The listing builds one solid part. Answer for the finished solid, in the listing's coordinates (mm). Give positions to 0.01 mm unless a question says otherwise; leave off trailing zeros. Order: outer loops, then holes, each group sorted by start corner. A loop starts at its lowest first (then second) coordinate and runs counter-clockwise, first axis right, second up.
```python
from build123d import *

# Parameters (mm, degrees)
ESBO_O1_W                = 152
ESBO_O1_H                = 60
RESSALTO_EXTRUS_O2_DEPTH = 6


with BuildPart() as part:
    # Esboço1 → Ressalto-extrusão2 (new body)
    with BuildSketch(Plane.XY):
        Rectangle(ESBO_O1_W, ESBO_O1_H)
        with BuildLine():
            Line((45, -16), (-45, -16))
            ThreePointArc((-45, -16), (-52.071067812, -13.071067812), (-55, -6))
            Line((-55, -6), (-55, 6))
            ThreePointArc((-55, 6), (-52.071067812, 13.071067812), (-45, 16))
            Line((-45, 16), (45, 16))
            ThreePointArc((45, 16), (52.071067812, 13.071067812), (55, 6))
            Line((55, 6), (55, -6))
            ThreePointArc((55, -6), (52.071067812, -13.071067812), (45, -16))
        make_face(mode=Mode.SUBTRACT)
    extrude(amount=RESSALTO_EXTRUS_O2_DEPTH)


solid = part.part
```
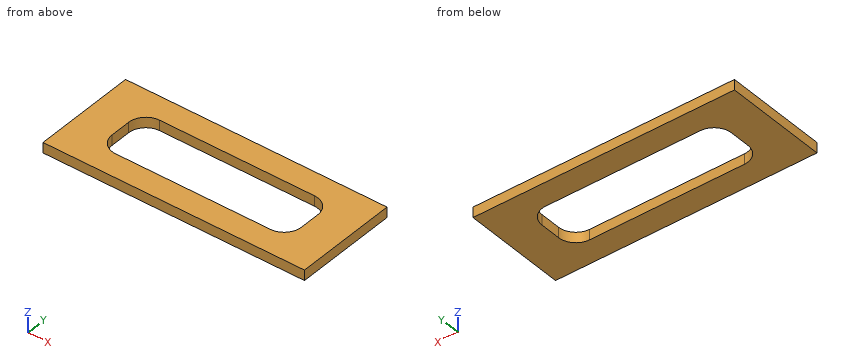
1) Find section C-C (x = 35.5). Write down the section's boundary in (y, z).
Geometry says:
outline: (-30, 0) - (-16, 0) - (-16, 6) - (-30, 6) - close; (16, 0) - (30, 0) - (30, 6) - (16, 6) - close
2) Find section B-B (y = -12). Write down the section's boundary in (x, z), then the cut area to 3 significant figures.
Geometry says:
outline: (-76, 0) - (-53, 0) - (-53, 6) - (-76, 6) - close; (53, 0) - (76, 0) - (76, 6) - (53, 6) - close
area: 276 mm2
3) Straight lines are drawn through the part: probe 1 along Y at (x, z) = (-28.5, 5.65); probe 2 along X at (y, z) = (-4, 4.35); probe 3 along X at (y, z) = (-8, 5.8). For each, find the intervals that lie inside material, in ascending order.
Geometry says:
probe 1: y = -30 to -16, 16 to 30
probe 2: x = -76 to -55, 55 to 76
probe 3: x = -76 to -54.8, 54.8 to 76
4) Find section A-A (z = 4.6). Write down the section's boundary in (x, y).
Geometry says:
outline: (-76, -30) - (76, -30) - (76, 30) - (-76, 30) - close; hole (-55, -6) arc R10 ccw to (-45, -16) - (45, -16) arc R10 ccw to (55, -6) - (55, 6) arc R10 ccw to (45, 16) - (-45, 16) arc R10 ccw to (-55, 6) - close
